Here's how the part is built. I have some questions about the finished solid (model axes, mm). Face numbers are marked on the shaded views. A direction names the side the tool comes from. Give positions to 0.01 mm unless a question says otherwise; leave off trailing zeros. Loops run counter-clockwise (first coordinate to the right, second up) from the corner with the lowest first, then second, coordinate; pieces in that order, holes last.
Q1. If we section it at B-B (x = -222): Please give me the cut outline in (y, z), plus the area to 3 significant figures.
Q2. Will these pins go through, and if not, where does the flat tip stop? P1, Ø1, axis at x = 126.5, z = -105.5, coming from the -Y side; P2, Ø1, axis at y = -171, z = -137, coming from the +X side; P3, Ø8, axis at y = -100.5, z = -25, coming from the +X side; P4, Ø20.5, axis at x = -215.97, z = -122.11, coming from the -Y side.
Q3. If we section it at C-C (y = -260.5): Please give me the cut outline in (x, z).
Q4. I need wall thicknesses on line 1 (X direction, y = -40.5, z = -115); line 2 (Y direction, x = 35, z = -54); line 3 (Z direction, x = -122, y = -69). Which ranges of each line are inside material? Lowest first, please.
Q5. For the marked faces 5, 6 and 7, which set-ups out of +Z, -Z, +X, -X, +Y, -Y let a thin tool reach every point of the face, with its end or its side?
Q6. We'd pull the mould along X, two halves only. Please class the marked faces 1, 2, 3 and 4: +X half, -X half, draft (parallel to the pull), parting line (faces both ways), or undercut.
Q7. If we section it at D-D (y = -158.5): Please give me the cut outline in (x, z).
Q8. If we section it at A-A (z = -129): Please give me the cut outline in (x, y).
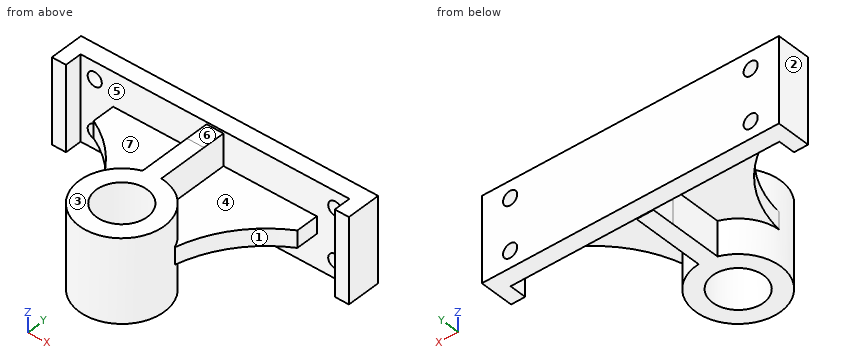
from build123d import *

# Parameters (mm, degrees)
BOSS_EXTRUDE1_DEPTH  = 152.4
SKETCH3_R            = 12.7
CUT_EXTRUDE1_DEPTH   = 40.64
BOSS_EXTRUDE2_DEPTH  = 40.64
BOSS_EXTRUDE7_DEPTH  = 30.48
SKETCH5_16_R         = 45.72
BOSS_EXTRUDE9_DEPTH  = 92.456
SKETCH9_W            = 206.074408616
SKETCH9_H            = 47.358127706
CUT_EXTRUDE3_DEPTH   = 256.032
SKETCH10_W           = 15.17458933
SKETCH10_H           = 40.64
BOSS_EXTRUDE10_DEPTH = 61.976
SKETCH11_W           = 15.24
SKETCH11_H           = 40.64
BOSS_EXTRUDE11_DEPTH = 56.934608


with BuildPart() as part:
    # Sketch1 → Boss-Extrude1 (new body)
    with BuildSketch(Plane.XY):
        Polygon((266.7, 15.24), (-266.7, 15.24), (-266.7, -15.24), (-266.7, -45.72), (-241.3, -45.72), (-241.3, -15.24), (241.3, -15.24), (241.3, -45.72), (266.7, -45.72), (266.7, -15.24), align=None)
    extrude(amount=-BOSS_EXTRUDE1_DEPTH)

    # Sketch3 → Cut-Extrude1 (cut)
    with BuildSketch(Plane(origin=(0, 15.24, 0), x_dir=(1, 0, 0), z_dir=(0, 1, 0))):
        with Locations(Location((215.972235605, 122.105743834, 0), (0, 0, 270))):
            Circle(SKETCH3_R)
        with Locations(Location((215.972235605, 30.414369603, 0), (0, 0, 270))):
            Circle(SKETCH3_R)
        with Locations(Location((-215.972235605, 122.105743834, 0), (0, 0, 270))):
            Circle(SKETCH3_R)
        with Locations(Location((-215.972235605, 30.414369603, 0), (0, 0, 270))):
            Circle(SKETCH3_R)
    extrude(amount=-CUT_EXTRUDE1_DEPTH, mode=Mode.SUBTRACT)

    # Sketch4 → Boss-Extrude2 (add)
    with BuildSketch(Plane.XZ.offset(15.24)):
        Polygon((-182.88, -60.96), (-182.88, -91.44), (0, -91.44), (0, -76.2), (0, -60.96), align=None)
        Polygon((0, -76.2), (0, -91.44), (182.88, -91.44), (182.88, -60.96), (0, -60.96), align=None)
    extrude(amount=BOSS_EXTRUDE2_DEPTH)

    # Sketch5 → Boss-Extrude7 (add)
    with BuildSketch(Plane.XY.offset(-60.96)):
        with BuildLine():
            Line((-15.24, -148.839934257), (-15.24, -55.88))
            Line((-15.24, -55.88), (-76.2, -55.88))
            Line((-76.2, -55.88), (-182.88, -55.88))
            ThreePointArc((-182.88, -55.88), (-104.636686401, -122.326673794), (-66.442758058, -217.60731411))
            ThreePointArc((-66.442758058, -217.60731411), (-51.430319931, -175.339319441), (-15.24, -148.839934257))
        make_face()
        with BuildLine():
            Line((182.88, -55.88), (15.24, -55.88))
            Line((15.24, -55.88), (15.24, -144.84950765))
            ThreePointArc((15.24, -144.84950765), (54.663389815, -159.335335359), (80.423000783, -192.508898804))
            ThreePointArc((80.423000783, -192.508898804), (117.142790659, -113.314475438), (182.88, -55.88))
        make_face()
    extrude(amount=-BOSS_EXTRUDE7_DEPTH)

    # Sketch5_16 → Boss-Extrude9 (add, symmetric)
    with BuildSketch(Plane.XY.offset(-60.96)):
        with BuildLine():
            Line((-15.24, -55.88), (15.24, -55.88))
            Line((15.24, -55.88), (15.24, -144.84950765))
            ThreePointArc((15.24, -144.84950765), (19.579997786, -296.402247336), (-15.24, -148.839934257))
            Line((-15.24, -148.839934257), (-15.24, -55.88))
        make_face()
        with Locations(Location((9.688342188, -220.847001658, 0), (0, 0, 180))):
            Circle(SKETCH5_16_R, mode=Mode.SUBTRACT)
    extrude(amount=BOSS_EXTRUDE9_DEPTH, both=True)

    # Sketch9 → Cut-Extrude3 (cut)
    with BuildSketch(Plane(origin=(0, -55.88, 0), x_dir=(1, 0, 0), z_dir=(0, 1, 0))):
        with Locations((3.259772677, -19.655003422)):
            Rectangle(SKETCH9_W, SKETCH9_H)
    extrude(amount=-CUT_EXTRUDE3_DEPTH, mode=Mode.SUBTRACT)

    # Sketch10 → Boss-Extrude10 (add)
    with BuildSketch(Plane(origin=(0, 0, -91.44), x_dir=(-1, 0, 0), z_dir=(0, 0, -1))):
        with Locations((-7.587294665, -35.56)):
            Rectangle(SKETCH10_W, SKETCH10_H)
        with Locations((7.587294665, -35.56)):
            Rectangle(SKETCH10_W, SKETCH10_H)
    extrude(amount=BOSS_EXTRUDE10_DEPTH)

    # Sketch11 → Boss-Extrude11 (add)
    with BuildSketch(Plane.XY.offset(-60.96)):
        with Locations((-7.62, -35.56)):
            Rectangle(SKETCH11_W, SKETCH11_H)
        with Locations((7.62, -35.56)):
            Rectangle(SKETCH11_W, SKETCH11_H)
    extrude(amount=BOSS_EXTRUDE11_DEPTH)


solid = part.part
Check sheet entries:
1. outline: (-15.24, -152.4) - (15.24, -152.4) - (15.24, -133.28) - (-15.24, -133.28) - close; (-15.24, -110.93) - (15.24, -110.93) - (15.24, -41.59) - (-15.24, -41.59) - close; (-15.24, -19.24) - (15.24, -19.24) - (15.24, 0) - (-15.24, 0) - close
1. area: 3,280 mm2
2. P1: stops at y = -15.24
2. P2: stops at x = 67.75
2. P3: stops at x = 15.24
2. P4: passes through
3. outline: (-55.38, -153.42) - (-13.07, -153.42) - (-13.07, -4.02) - (-55.38, -4.02) - close; (32.45, -153.42) - (74.76, -153.42) - (74.76, -4.02) - (32.45, -4.02) - close
4. line 1: x = -266.7 to -241.3, -15.17 to 15.17, 241.3 to 266.7
4. line 2: y = -292.72 to -258.92, -182.77 to -148.97, -15.24 to 15.24
4. line 3: z = -91.44 to -60.96
5. face 5: none
5. face 6: +Z, -Y
5. face 7: +Z
6. face 1: +X half
6. face 2: -X half
6. face 3: draft
6. face 4: undercut
7. outline: (-83.64, -91.44) - (-34.12, -91.44) - (-34.12, -153.42) - (53.5, -153.42) - (53.5, -91.44) - (91.32, -91.44) - (91.32, -60.96) - (53.5, -60.96) - (53.5, -4.02) - (-34.12, -4.02) - (-34.12, -60.96) - (-83.64, -60.96) - close
8. outline: (-266.7, -45.72) - (-241.3, -45.72) - (-241.3, -15.24) - (-226.64, -15.24) - (-226.64, 15.24) - (-266.7, 15.24) - close; (-205.31, -15.24) - (-15.17, -15.24) - (-15.17, -55.88) - (-15.24, -55.88) - (-15.24, -148.84) arc R76.2 ccw (long way) to (15.24, -144.85) - (15.24, -55.88) - (15.17, -55.88) - (15.17, -15.24) - (205.31, -15.24) - (205.31, 15.24) - (-205.31, 15.24) - close; (226.64, -15.24) - (241.3, -15.24) - (241.3, -45.72) - (266.7, -45.72) - (266.7, 15.24) - (226.64, 15.24) - close; hole circle Ø91.44 at (9.69, -220.85)
